For this review, take the finished solid that the model builds, in its own axes (mm). A direction names the side the tool comes from. Round coordinates to 2 decimals unless told otherwise and drop trailing zeros. Answer in a Markdown table with one row per item. Add a question column.
from build123d import *

# Parameters (mm, degrees)
F1_DEPTH = 25
F1_TAPER = -2
F2_R     = 6
F3_T     = 3
F5_D     = 10


# Not quite as in the source:
# - a shell that OpenCascade refuses in one call is made with other operations: the cavity is built on its own and cut out


with BuildPart() as f1:
    # F0 (on Top) → F1 (new body)
    with BuildSketch(Plane.XY):
        with BuildLine():
            Line((55, 25), (0, 25))
            ThreePointArc((0, 25), (-17.6776695297, 17.6776695297), (-25, 0))
            Line((-25, 0), (-25, -25))
            ThreePointArc((-25, -25), (-22.0710678119, -32.0710678119), (-15, -35))
            Line((-15, -35), (45, -35))
            ThreePointArc((45, -35), (52.0710678119, -32.0710678119), (55, -25))
            Line((55, -25), (55, 25))
        make_face()
    extrude(amount=F1_DEPTH, taper=F1_TAPER)

    # F2
    f2_edges = [f1.edges().sort_by_distance(p)[0] for p in [
        (15, -35.873019, 25),
    ]]
    fillet(f2_edges, radius=F2_R)

    # F3: shell of thickness 3, made by hand


with BuildPart() as f3_core1:
    # F3_t2: copy of F1
    add(f1.part)

    # the walls: a layer under each face that stays
    f3_faces = [f3_core1.faces().sort_by_distance(p)[0] for p in [
        (27.6640479465, 25.328095893, 9.3954370929),
        (-17.9096696286, 17.9096696286, 9.395488449),
        (27.794131329, 23.9760199568, 23.1679440438),
        (15, -5, 0),
        (55.3280962996, 0.1640481498, 9.3954487356),
        (-25.3280911583, -12.5, 9.3953015099),
        (-16.9638078754, 16.9431979233, 23.1679501064),
        (53.9760549891, 0.2869115749, 23.1679425379),
        (-22.3030632948, -32.3030632948, 9.3953015099),
        (15, -35.3280911583, 9.3953015099),
        (52.3030694739, -32.3030694739, 9.3955517523),
        (-23.9758761566, -12.5, 23.1679502228),
        (51.3377505062, -31.3560472609, 23.1679500628),
        (15, -33.9758761566, 23.1679502228),
        (-21.3469028974, -31.3469028974, 23.1679502228),
    ]]
    thicken(f3_faces, amount=-F3_T, mode=Mode.SUBTRACT)


with BuildPart() as f1_1:
    add(f1.part)

    # what is left inside the walls is the cavity
    f3_cavity = [f3_core1.part.solids().sort_by_distance(p)[0] for p in [
        (27.367645, -5, 3.03),
    ]]
    add(f3_cavity, mode=Mode.SUBTRACT)

    # F5 (through all)
    with Locations(Plane(origin=(54.9330113821, 0, -1.918303028), x_dir=(0, 1, 0), z_dir=(0.999390827, 0, -0.0348994967))):
        with Locations((0, 8.7753692642)):
            Hole(F5_D / 2)


solid = f1_1.part
Q1. Tool access review of faces 1 (the face through (49.66, -3, 24)), 2 (the face through (-20.28, -30.16, 11.06)), 3 (the face through (-22.386, -32.226, 9.527)): name each direction out of +Z, -Z, +X, -X, +Y, -Y from which nothing blocks a thin tool from reaching the whole face with its end or side.
Q2. Insertion check: pin 1 Ø6 at (x, y) = (14, -22.5) entering from +Z; pin 2 Ø3.5 at (x, z) = (14, 23) entering from +Y; pin 3 Ø5 at (y, z) = (-6, 10) entering from +X. Each pin has a flat end and moves straight along its axis. Give the tip position at first contact, or say it passes through.
Q3. To check wall thickness, follow probe 1 along Z at (x, y) = (16, -3); probe 2 along Y at (x, z) = (16, 8.75); probe 3 along Y at (x, z) = (50.5, 20.75). State the ranges of each line that lie inside material, in increasing order.
Q4. Add section A-A on y = 1.5. Count the separate pieces of the cut face and the enclosed holes in it, then the cut area to 3 significant figures.
Q5. Draft analysis for pull direction Y (two halves, no side actions). For faces 4 (the face through (-17.715, 18.109, 9.527)), 5 (the face through (-23.607, 3.685, 12.986)), 6 (the face through (52.226, -32.386, 9.527)), state which applies: released by +Y, released by -Y, zero draft, split by the parting line, or undercut.
Answer sheet:
| question | item | result |
|---|---|---|
| 1 | face 1 | +Z |
| 1 | face 2 | none |
| 1 | face 3 | -Z, -X, -Y |
| 2 | pin 1 | stops at z = 3 |
| 2 | pin 2 | stops at y = 25.22 |
| 2 | pin 3 | stops at x = 55.44 |
| 3 | probe 1 | z = 0 to 3 |
| 3 | probe 2 | y = -35.31 to -32.3, 22.3 to 25.31 |
| 3 | probe 3 | y = -33.83 to -29.48, 22.1 to 25.4 |
| 4 | separate pieces | 3 |
| 4 | enclosed holes | 0 |
| 4 | area | 312 mm² |
| 5 | face 4 | released by +Y |
| 5 | face 5 | undercut |
| 5 | face 6 | released by -Y |
